For this review, take the finished solid that the model builds, in its own axes (mm). A direction names the side the tool comes from. Round coordinates to 2 decimals unless told otherwise and drop trailing zeros. Write each loop counter-clockwise with the first axis right and the second up, starting at its lowest first coordinate (ties: lowest second). Pieces come first, ordered by that corner, then holes. Notation, with made-up numbers: M -14.5,20 L 30.5,20 A28 cw 30.5,39 Z; hole C 4,42.25 d2. An arc over 180 degrees is marked long. Answer in a Markdown table with one row per item.
```python
from build123d import *

# Parameters (mm, degrees)
BOSS_EXTRUDE1_DEPTH = 6.35
CAVITY1_START       = 298.45
CAVITY1_OUTLINE_R   = 12.7
CAVITY1_DEPTH       = 12.7
CAVITY1_START_2     = 720.91620239
CAVITY1_2_DEPTH     = 22.43918751
SKETCH2_W           = 22.270177668
SKETCH2_H           = 113.672619585
CUT_EXTRUDE1_DEPTH  = 1143.349273427


# Read off the part's stored shape, not the designer's step: Cavity1
with BuildPart() as part:
    # Sketch1 → Boss-Extrude1 (new, symmetric)
    with BuildSketch(Plane(origin=(0, 304.8, 0), x_dir=(1, 0, 0), z_dir=(0, 1, 0))):
        Polygon((798.4, -133.35), (1001.6, -133.35), (1001.6, -260.35), (1014.3, -260.35), (1014.3, -133.35), (1065.1, -133.35), (1065.1, -412.75), (1014.3, -412.75), (1001.6, -412.75), (798.4, -412.75), (785.7, -412.75), (734.9, -412.75), (734.9, -133.35), (785.7, -133.35), (785.7, -260.35), (798.4, -260.35), align=None)
    extrude(amount=BOSS_EXTRUDE1_DEPTH, both=True)

    # Cavity1 outline → Cavity1 (cut)
    with BuildSketch(Plane(origin=(0, 0, 0), x_dir=(1, 0, 0), z_dir=(0, 1, 0)).offset(CAVITY1_START)):
        with Locations((900, -250)):
            Circle(CAVITY1_OUTLINE_R)
    extrude(amount=CAVITY1_DEPTH, mode=Mode.SUBTRACT)

    # Cavity1 2 outline → Cavity1 2 (cut)
    with BuildSketch(Plane(origin=(0, 0, 0), x_dir=(0.7149295353100829, -0.698752516444498, 0.02491345627949748), z_dir=(0.6991965099607612, 0.7144755512387372, -0.025474048378572107)).offset(CAVITY1_START_2)):
        with BuildLine():
            Line((312, -255.374549574), (314.076314529, -255.435688643))
            ThreePointArc((314.076314529, -255.435688643), (327.146171675, -242.424687318), (313.444242413, -230.081087528))
            Line((313.444242413, -230.081087528), (312, -230.195835843))
            Line((312, -230.195835843), (312, -255.374549574))
        make_face()
    extrude(amount=CAVITY1_2_DEPTH, mode=Mode.SUBTRACT)

    # Sketch2 → Cut-Extrude1 (cut, through all)
    with BuildSketch(Plane(origin=(0, 311.15, 0), x_dir=(1, 0, 0), z_dir=(0, 1, 0))):
        with Locations((746.035088834, -190.186309793)):
            Rectangle(SKETCH2_W, SKETCH2_H)
    extrude(amount=-CUT_EXTRUDE1_DEPTH, mode=Mode.SUBTRACT)


solid = part.part
```
Q1. Take a section at B-B (y = 303). State the section outline as (x, z) points.
Found:
| item | result |
|---|---|
| outline | M 734.9,247.02 L 757.17,247.02 L 757.17,133.35 L 785.7,133.35 L 785.7,260.35 L 798.4,260.35 L 798.4,133.35 L 1001.6,133.35 L 1001.6,260.35 L 1014.3,260.35 L 1014.3,133.35 L 1065.1,133.35 L 1065.1,412.75 L 734.9,412.75 Z; hole C 900,250 d25.4 |
Q2. Mouldability with a two-part tool opening along X and no side actions: class faces 1 (the face through (785.7, 305, 196)), 2 (the face through (734.9, 305, 331)), 3 (the face through (902, 311.15, 271)), 4 (the face through (1065.1, 305, 271)) as +X half, -X half, draft (parallel to the pull), parting line (faces both ways), or undercut.
Found:
| item | result |
|---|---|
| face 1 | undercut |
| face 2 | -X half |
| face 3 | draft |
| face 4 | +X half |
Q3. Machinability: for faces 5 (the face through (798.4, 305, 198)), 6 (the face through (899, 305, 133.35)), 7 (the face through (746, 305, 247.023)), which of the approach directions +Z, -Z, +X, -X, +Y, -Y give a long, thin tool a straight path to every point of the face, cutting with its end or side? Answer none if there is none.
Found:
| item | result |
|---|---|
| face 5 | -Z, +Y, -Y |
| face 6 | -Z, +X, -X, +Y, -Y |
| face 7 | -Z, -X, +Y, -Y |
Q4. For probe 1 along X at (y, z) = (301.75, 250); probe 2 along X at (y, z) = (310.25, 232); probe 3 along Z at (x, y) = (899.5, 300), list the stretches that pass through material, from the lowest coordinate up.
Found:
| item | result |
|---|---|
| probe 1 | 734.9 to 785.7, 798.4 to 887.3, 912.7 to 1001.6, 1014.3 to 1065.1 |
| probe 2 | 757.17 to 785.7, 798.4 to 1001.6, 1014.3 to 1065.1 |
| probe 3 | 133.35 to 237.31, 262.69 to 412.75 |
Q5. Insertion check: P1, Ø4, axis at y = 305, z = 173.5, coming from the -X side; P2, Ø20.5, axis at x = 900, z = 250, coming from the +Y side; P3, Ø6.5, axis at x = 1006.5, y = 304, coming from the -Z side. Each pin has a flat end and moves straight along its axis. Give the tip position at first contact, or say it passes through.
Found:
| item | result |
|---|---|
| P1 | x = 757.17 |
| P2 | through |
| P3 | z = 260.35 |
Q6. Take a section at C-C (z = 254). State the section outline as (x, y) points, then the cut area to 3 significant figures.
Found:
| item | result |
|---|---|
| outline | M 734.9,298.45 L 785.7,298.45 L 785.7,311.15 L 734.9,311.15 Z; M 798.4,298.45 L 887.95,298.45 L 887.95,311.15 L 798.4,311.15 Z; M 912.05,298.45 L 1001.6,298.45 L 1001.6,311.15 L 912.05,311.15 Z; M 1014.3,298.45 L 1065.1,298.45 L 1065.1,311.15 L 1014.3,311.15 Z |
| area | 3,560 mm² |
Q7. Take a section at A-A (x = 900). State the section outline as (y, z) points.
Found:
| item | result |
|---|---|
| outline | M 298.45,133.35 L 311.15,133.35 L 311.15,237.3 L 298.45,237.3 Z; M 298.45,262.7 L 311.15,262.7 L 311.15,412.75 L 298.45,412.75 Z |
